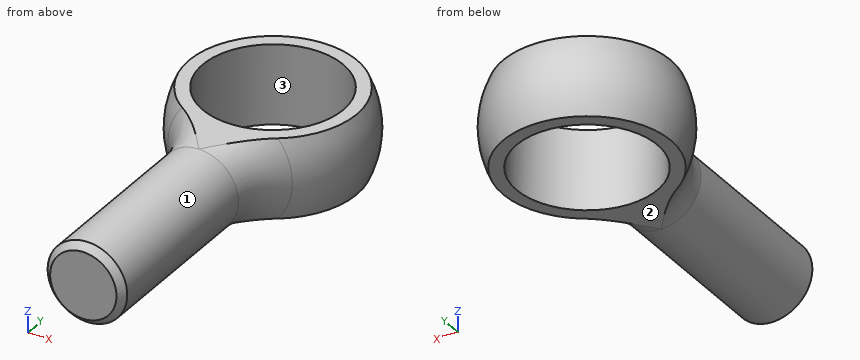
```python
from build123d import *

# Parameters (mm, degrees)
SKETCH1_W               = 9.525
SKETCH1_H               = 44.45
CHAMFER2_SIZE           = 1.5875
CUT_EXTRUDE1_DEPTH      = 60.737268518
CUT_EXTRUDE1_DEPTH_BACK = 60.737268518
SKETCH5_W               = 12.7
SKETCH5_H               = 50.8
CUT_EXTRUDE2_DEPTH      = 57.261143358
CUT_EXTRUDE2_DEPTH_BACK = 57.261143358
SKETCH6_R               = 16.8354375
CUT_EXTRUDE3_DEPTH      = 58.900240514
CUT_EXTRUDE3_DEPTH_BACK = 58.900240514
SKETCH8_W               = 11.1125
SKETCH8_H               = 50.8
CUT_EXTRUDE4_DEPTH      = 58.900240514
CUT_EXTRUDE4_DEPTH_BACK = 58.900240514
SKETCH10_R              = 9.525
CHAMFER1_SIZE           = 0.9525


with BuildPart() as part:
    # Sketch1 → Revolve1 (revolve)
    with BuildSketch(Plane.XY, mode=Mode.PRIVATE) as revolve1_sk:
        with Locations((4.7625, -22.225)):
            Rectangle(SKETCH1_W, SKETCH1_H)
    revolve(revolve1_sk.sketch.rotate(Axis((0, 50.8, 0), (0, -1, 0)), 180), axis=Axis((0, 50.8, 0), (0, -1, 0)))

    # Chamfer2
    chamfer2_edges = [part.edges().sort_by_distance(p)[0] for p in [
        (9.525, -44.45, 0),
    ]]
    chamfer(chamfer2_edges, length=CHAMFER2_SIZE)

    # Sketch4 → Revolve2 (revolve)
    with BuildSketch(Plane.XY):
        with BuildLine():
            Line((9.525, 0), (0, 0))
            Line((0, 0), (0, 50.8))
            ThreePointArc((0, 50.8), (20.743606098, 36.553310038), (14.893041237, 12.078092784))
            ThreePointArc((14.893041237, 12.078092784), (10.927447707, 6.608634352), (9.525, 0))
        make_face()
    revolve(axis=Axis((0, 50.8, 0), (0, 1, 0)))

    # Sketch5 → Cut-Extrude1 (cut, two sides: drawn at the far end of the back side and taken through both)
    with BuildSketch(Plane(origin=(0, 0, 0), x_dir=(0, 0, -1), z_dir=(1, 0, 0)).offset(-CUT_EXTRUDE1_DEPTH_BACK)):
        with Locations((15.875, 25.4)):
            Rectangle(SKETCH5_W, SKETCH5_H)
        with Locations((-15.875, 25.4)):
            Rectangle(SKETCH5_W, SKETCH5_H)
    extrude(amount=CUT_EXTRUDE1_DEPTH + CUT_EXTRUDE1_DEPTH_BACK, mode=Mode.SUBTRACT)

    # Sketch6 → Cut-Extrude2 (cut, two sides: drawn at the far end of the back side and taken through both)
    with BuildSketch(Plane.XY.offset(-CUT_EXTRUDE2_DEPTH_BACK)):
        with Locations((0, 28.575)):
            Circle(SKETCH6_R)
    extrude(amount=CUT_EXTRUDE2_DEPTH + CUT_EXTRUDE2_DEPTH_BACK, mode=Mode.SUBTRACT)


with BuildPart() as body_2:
    # Sketch7 → Revolve3 (revolve)
    with BuildSketch(Plane.XY):
        with BuildLine():
            Line((0, 45.24375), (0, 11.90625))
            ThreePointArc((0, 11.90625), (16.66875, 28.575), (0, 45.24375))
        make_face()
    revolve(axis=Axis((0, 0, 0), (0, 1, 0)))

    # Sketch8 → Cut-Extrude3 (cut, two sides: drawn at the far end of the back side and taken through both)
    with BuildSketch(Plane(origin=(0, 0, 0), x_dir=(0, 0, -1), z_dir=(1, 0, 0)).offset(-CUT_EXTRUDE3_DEPTH_BACK)):
        with Locations((-16.66875, 25.4)):
            Rectangle(SKETCH8_W, SKETCH8_H)
        with Locations((16.66875, 25.4)):
            Rectangle(SKETCH8_W, SKETCH8_H)
    extrude(amount=CUT_EXTRUDE3_DEPTH + CUT_EXTRUDE3_DEPTH_BACK, mode=Mode.SUBTRACT)

    # Sketch10 → Cut-Extrude4 (cut, two sides: drawn at the far end of the back side and taken through both)
    with BuildSketch(Plane.XY.offset(-CUT_EXTRUDE4_DEPTH_BACK)):
        with Locations((0, 28.575)):
            Circle(SKETCH10_R)
    extrude(amount=CUT_EXTRUDE4_DEPTH + CUT_EXTRUDE4_DEPTH_BACK, mode=Mode.SUBTRACT)

    # Chamfer1
    chamfer1_edges = [body_2.edges().sort_by_distance(p)[0] for p in [
        (-9.525, 28.575, -11.1125),
        (-9.525, 28.575, 11.1125),
    ]]
    chamfer(chamfer1_edges, length=CHAMFER1_SIZE)


solid = part.part
```
Geometry check sheet. Reference: the model listing, model coordinates, mm. Face numbers are marked on the shaded views. Coordinates: 2 decimals unless noted, no trailing zeros. Write each loop counter-clockwise with the first axis right and the second up, starting at its lowest first coordinate (ties: lowest second). Pieces come first, ordered by that corner, then holes. Notation, with made-up numbers: M -3.75,2 L 18.25,2 A15 cw 18.25,8 Z; hole C 12,-36.5 d3. An arc over 180 degrees is marked long. One line per item, written item: value. Start each with the question number.
(1) Sectioned sample at D-D, the plane x = -18.5. Enter the section's corners in (y, z) (3 decimals).
(2) Release check for a two-part mould opening along X. For the marked faces 1, 2 and 3 record: released by +X, released by -X, zero draft, split by the parting line, or undercut.
(3) Sectioned sample at C-C, the plane y = -15. Enter the section's corners in (x, z) (3 decimals), and give its area (3 significant figures).
(4) Depth check by flat-ended pin: pin 1 (20 mm diameter, centred on x = 0, y = 28.575, fed in from +Z); pin 2 (2 mm diameter, centred on x = 5.5, y = -18.5, fed in from -Z) (3 decimals); pin 3 (5 mm diameter, centred on y = -17.5, z = 3, fed in from -X); pin 4 (1.5 mm diameter, centred on y = 4, z = -1.5, fed in from +X). Enter the tip coordinate at first touch or a pass-through.
(5) Scan lines: line 1 along Y through (x, z) = (0, 0); line 2 along X through (y, z) = (28, 3.25); line 3 along Y through (x, z) = (9, 6). Record each from-to range of solid material in increasing order. Write a range as [from, to].
(6) Sectioned sample at A-A, the plane y = 37. Enter the section's corners in (x, z) (3 decimals).
Filled sheet:
1. outline: M 20.766,-9.525 L 36.384,-9.525 A12.317 ccw 36.384,9.525 L 20.766,9.525 A12.317 ccw Z
2. face 1: split by the parting line
2. face 2: zero draft
2. face 3: undercut
3. outline: C 0,0 d19.05
3. area: 285 mm²
4. pin 1: through
4. pin 2: z = -8.395
4. pin 3: x = -9.51
4. pin 4: x = 10.14
5. line 1: [-44.45, 11.74], [45.41, 50.8]
5. line 2: [-21.98, -16.83], [16.83, 21.98]
5. line 3: [6.35, 14.35], [42.8, 47.99]
6. outline: M -18.228,-9.525 L -14.576,-9.525 L -14.576,9.525 L -18.228,9.525 A20.566 ccw Z; M 14.576,-9.525 L 18.228,-9.525 A20.566 ccw 18.228,9.525 L 14.576,9.525 Z
